Source: CAD feature listing. Evaluate the final solid. Frame: model axes, mm. A direction names the side the tool comes from. Round coordinates to 2 decimals unless told otherwise and drop trailing zeros. Order: outer loops, then holes, each group sorted by start corner. A loop starts at its lowest first (then second) coordinate and runs counter-clockwise, first axis right, second up. Notation, with made-up numbers: (-28.75, 43.25) - (-6.75, 43.25) arc R23 cw to (-6.75, 74.25) - close; hole circle Ø6 at (23, -6). An arc over 180 degrees is marked (long way). Put each result on its own line as item: value. Start each with the question number.
1) Line query: probe 1 along X at (y, z) = (0.95, -15); probe 2 along Z at (x, y) = (-4, 4.6); probe 3 along X at (y, z) = (0.55, -14). Output: solid intervals per line, ascending. Write a range as [from, to].
2) Section C-C on y = 1.1. Output: boundary loops of the cut face in (x, z), then the cut area to 3 significant figures.
3) Contact query for flat-ended pins moving along their axis: P1, Ø2, axis at x = -8, z = 15, coming from the -Y side; P2, Ø2, axis at x = 11.5, z = -3.5, coming from the -Y side; P3, Ø7.5, axis at x = -4, z = 13.5, coming from the +Y side. Output: stop coordinate, or through.
4) Section A-A on z = 15. Output: boundary loops of the cut face in (x, y).
5) Access query for faces 1 (the face through (0, 2, 14)), 2 (the face through (0, 2, -18.5)), 3 (the face through (11, 2, 0)). Directions: +Z, -Z, +X, -X, +Y, -Y. A direction counts if a zero-diameter tool reaches every point of the face in a straight line with its end or side. Return the directions, or none.
6) Mould query, pull axis X, two halves, no side actions, for faces 4 (the face through (0, 2, 18.5)), 5 (the face through (12.25, 3, 0)), 6 (the face through (7.33, 0.99, 15.87)). Classes: +X half, -X half, draft (parallel to the pull), parting line (faces both ways), or undercut.
7) Section B-B on x = 8. Output: boundary loops of the cut face in (y, z), then the cut area to 3 significant figures.
8) Section D-D on x = -4.5. Output: boundary loops of the cut face in (y, z), then the cut area to 3 significant figures.
```python
from build123d import *

# Parameters (mm, degrees)
SKETCH_1_W          = 20.5
SKETCH_1_H          = 35
EXTRUDE_1_DEPTH     = 2
SKETCH_2_W          = 24.5
SKETCH_2_H          = 37
SKETCH_2_W_2        = 20.5
SKETCH_2_H_2        = 35
EXTRUDE_2_DEPTH     = 5
SKETCH_3_R          = 1.1
CUT_EXTRUDE_1_DEPTH = 23.744504831
SKETCH_4_W          = 24.5
SKETCH_4_H          = 21.5
CUT_EXTRUDE_4_DEPTH = 2


with BuildPart() as part:
    # 草图1 → 凸台-拉伸1 (new body)
    with BuildSketch(Plane(origin=(0, 0, 0), x_dir=(1, 0, 0), z_dir=(0, 1, 0))):
        Rectangle(SKETCH_1_W, SKETCH_1_H)
    extrude(amount=EXTRUDE_1_DEPTH)

    # 草图2 → 凸台-拉伸2 (add)
    with BuildSketch(Plane(origin=(0, 0, 0), x_dir=(1, 0, 0), z_dir=(0, 1, 0))):
        Rectangle(SKETCH_2_W, SKETCH_2_H)
        Rectangle(SKETCH_2_W_2, SKETCH_2_H_2, mode=Mode.SUBTRACT)
    extrude(amount=EXTRUDE_2_DEPTH)

    # 草图3 → 切除-拉伸1 (cut, through all)
    with BuildSketch(Plane.XZ):
        with Locations(Location((-8, 15, 0), (0, 0, 270))):
            Circle(SKETCH_3_R)
        with Locations(Location((8, 15, 0), (0, 0, 270))):
            Circle(SKETCH_3_R)
        with Locations(Location((8, -15, 0), (0, 0, 270))):
            Circle(SKETCH_3_R)
        with Locations(Location((-8, -15, 0), (0, 0, 270))):
            Circle(SKETCH_3_R)
    extrude(amount=-CUT_EXTRUDE_1_DEPTH, mode=Mode.SUBTRACT)

    # 草图4 → 切除-拉伸4 (cut)
    with BuildSketch(Plane.XZ):
        Rectangle(SKETCH_4_W, SKETCH_4_H)
    extrude(amount=-CUT_EXTRUDE_4_DEPTH, mode=Mode.SUBTRACT)


solid = part.part
```
Answer sheet:
1. probe 1: [-12.25, -9.1], [-6.9, 6.9], [9.1, 12.25]
1. probe 2: [-18.5, -17.5], [17.5, 18.5]
1. probe 3: [-12.25, -8.46], [-7.54, 7.54], [8.46, 12.25]
2. outline: (-12.25, -18.5) - (12.25, -18.5) - (12.25, -10.75) - (-12.25, -10.75) - close; (-12.25, 10.75) - (12.25, 10.75) - (12.25, 18.5) - (-12.25, 18.5) - close; hole circle Ø2.2 at (-8, -15); hole circle Ø2.2 at (-8, 15); hole circle Ø2.2 at (8, -15); hole circle Ø2.2 at (8, 15)
2. area: 365 mm^2
3. P1: through
3. P2: y = 2
3. P3: y = 2
4. outline: (-12.25, 0) - (-9.1, 0) - (-9.1, 2) - (-10.25, 2) - (-10.25, 5) - (-12.25, 5) - close; (-6.9, 0) - (6.9, 0) - (6.9, 2) - (-6.9, 2) - close; (9.1, 0) - (12.25, 0) - (12.25, 5) - (10.25, 5) - (10.25, 2) - (9.1, 2) - close
5. face 1: +Y
5. face 2: -Z, +X, -X, +Y, -Y
5. face 3: +X, -X, -Y
6. face 4: draft
6. face 5: +X half
6. face 6: undercut
7. outline: (0, -18.5) - (5, -18.5) - (5, -17.5) - (2, -17.5) - (2, -16.1) - (0, -16.1) - close; (0, -13.9) - (2, -13.9) - (2, -10.75) - (0, -10.75) - close; (0, 10.75) - (2, 10.75) - (2, 13.9) - (0, 13.9) - close; (0, 16.1) - (2, 16.1) - (2, 17.5) - (5, 17.5) - (5, 18.5) - (0, 18.5) - close
7. area: 28.2 mm^2
8. outline: (0, -18.5) - (5, -18.5) - (5, -17.5) - (2, -17.5) - (2, -10.75) - (0, -10.75) - close; (0, 10.75) - (2, 10.75) - (2, 17.5) - (5, 17.5) - (5, 18.5) - (0, 18.5) - close
8. area: 37.0 mm^2
